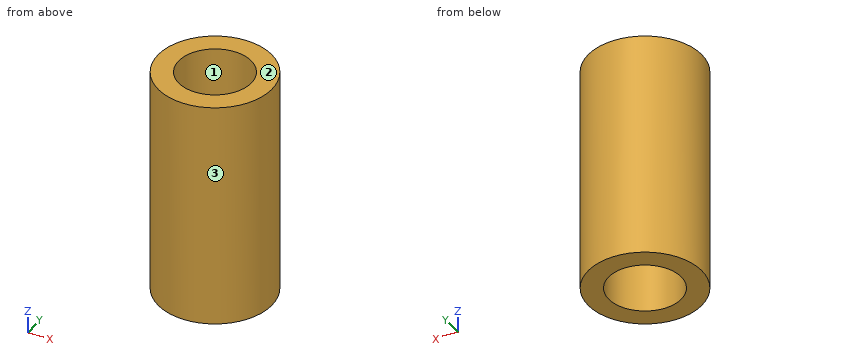
```python
from build123d import *

# Parameters (mm, degrees)
SKETCH059_R  = 1.6
PAD025_DEPTH = 10
SKETCH058_R  = 2.5
PAD024_DEPTH = 10


with BuildPart() as pad025:
    # Sketch059 → Pad025 (new body)
    with BuildSketch(Plane.XY.offset(10)):
        Circle(SKETCH059_R)
    extrude(amount=-PAD025_DEPTH)


with BuildPart() as cut040:
    # Sketch058 → Pad024 (new body)
    with BuildSketch(Plane.XY):
        Circle(SKETCH058_R)
    extrude(amount=PAD024_DEPTH)

    # Cut040: cut Pad025
    add(pad025.part, mode=Mode.SUBTRACT)


with BuildPart() as cut040_1:
    # Cut040 placement: moved
    add(cut040.part.moved(Location((37.5, -75.5, -88))))


solid = cut040_1.part
```
Part model, mm, in its own coordinate system. Face numbers are marked on the shaded views. Round coordinates to 2 decimals unless told otherwise and drop trailing zeros. Order: outer loops, then holes, each group sorted by start corner. A loop starts at its lowest first (then second) coordinate and runs counter-clockwise, first axis right, second up. Notation, with made-up numbers: M -24,44.25 L -15,44.25 A31 ccw -15,79.25 Z; hole C 2,59.25 d7. An arc over 180 degrees is marked long. Answer in a Markdown table with one row per item. Add a question column.
Q1. Cut at A-A on y = -75.5. Give the cut face in (x, z).
Q2. Cut at C-C on z = -81. Give the cut face in (x, y).
Q3. Pin check, flat tips, straight feed: pin 1 (3 mm diameter, centred on x = 35.5, z = -84.5, fed in from -Y); pin 2 (3 mm diameter, centred on x = 37.5, y = -75.5, fed in from -Z). Stop position of each tip, or through.
Q4. Wall check: L1, parallel to Y at x = 37.5, z = -85.5; L2, parallel to X at y = -76.9, z = -87; L3, parallel to X at y = -74.7, z = -78.75. Give the ranges that are in metal, low to high. Write a range as from..to.
Q5. Mould opens along X. For the marked faces 1, 2 and 3 say: +X half, -X half, draft (parallel to the pull), parting line (faces both ways), or undercut.
Q6. Cut at D-D on y = -77.2. Give the cut face in (x, z).
Q7. Cut at B-B on x = 37.5. Give the cut face in (y, z), and give its area (3 significant figures).
Established:
| question | item | result |
|---|---|---|
| 1 | outline | M 35,-88 L 35.9,-88 L 35.9,-78 L 35,-78 Z; M 39.1,-88 L 40,-88 L 40,-78 L 39.1,-78 Z |
| 2 | outline | C 37.5,-75.5 d5; hole C 37.5,-75.5 d3.2 |
| 3 | pin 1 | stops at y = -77.95 |
| 3 | pin 2 | passes through |
| 4 | L1 | y = -78..-77.1, -73.9..-73 |
| 4 | L2 | x = 35.43..36.73, 38.27..39.57 |
| 4 | L3 | x = 35.13..36.11, 38.89..39.87 |
| 5 | face 1 | undercut |
| 5 | face 2 | draft |
| 5 | face 3 | parting line |
| 6 | outline | M 35.67,-88 L 39.33,-88 L 39.33,-78 L 35.67,-78 Z |
| 7 | outline | M -78,-88 L -77.1,-88 L -77.1,-78 L -78,-78 Z; M -73.9,-88 L -73,-88 L -73,-78 L -73.9,-78 Z |
| 7 | area | 18.0 mm2 |
